The listing builds one solid part. Answer for the finished solid, in the listing's coordinates (mm). Face numbers are marked on the shaded views. A direction names the side the tool comes from. Give positions to 0.01 mm unless a question says otherwise; leave off trailing zeros. Write each loop counter-clockwise with the first axis right and the second up, starting at its lowest first coordinate (ties: lowest second). Pieces come first, ordered by that corner, then holes. Notation, with made-up numbers: (9.5, -39.75) - (36.5, -39.75) arc R15 ccw to (36.5, -10.75) - close; hole circle Ø3 at (20.5, 11.5). An arc over 180 degrees is marked (long way). One line per item, written item: value. Start each with the question number.
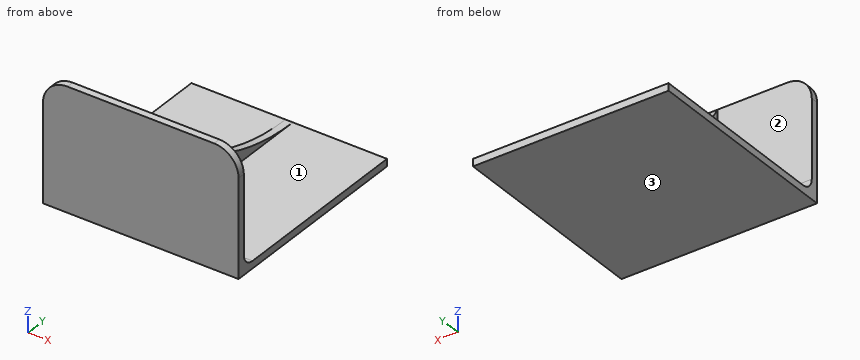
from build123d import *

# Parameters (mm, degrees)
SKETCH1_W           = 80
SKETCH1_H           = 50
BOSS_EXTRUDE1_DEPTH = 3
SKETCH2_W           = 80
SKETCH2_H           = 3
BOSS_EXTRUDE2_DEPTH = 82
BOSS_EXTRUDE3_DEPTH = 1.5
FILLET1_R           = 10
FILLET2_R           = 5


with BuildPart() as part:
    # Sketch1 → Boss-Extrude1 (new body)
    with BuildSketch(Plane(origin=(0, 0, 0), x_dir=(1, 0, 0), z_dir=(0, 1, 0))):
        Rectangle(SKETCH1_W, SKETCH1_H)
    extrude(amount=BOSS_EXTRUDE1_DEPTH)

    # Sketch2 → Boss-Extrude2 (add)
    with BuildSketch(Plane(origin=(0, 3, 0), x_dir=(1, 0, 0), z_dir=(0, 1, 0))):
        with Locations((0, 23.5)):
            Rectangle(SKETCH2_W, SKETCH2_H)
    extrude(amount=BOSS_EXTRUDE2_DEPTH)

    # Sketch3 → Boss-Extrude3 (add, symmetric)
    with BuildSketch(Plane(origin=(0, 0, 0), x_dir=(0, 0, -1), z_dir=(1, 0, 0))):
        with BuildLine():
            Line((22, 85), (22, 3))
            Line((22, 3), (-25, 3))
            ThreePointArc((-25, 3), (9.416947126, 37.742725428), (22, 85))
        make_face()
    extrude(amount=BOSS_EXTRUDE3_DEPTH, both=True)

    # Fillet1
    fillet1_edges = [part.edges().sort_by_distance(p)[0] for p in [
        (40, 1.5, 25),
        (-40, 1.5, 25),
    ]]
    fillet(fillet1_edges, radius=FILLET1_R)

    # Fillet2
    fillet2_edges = [part.edges().sort_by_distance(p)[0] for p in [
        (-20.75, 3, -22),
        (20.75, 3, -22),
    ]]
    fillet(fillet2_edges, radius=FILLET2_R)


solid = part.part
Item 1: Find section C-C on z = -9. Determine the outline of the cut face in (x, y).
Item 2: Each of these flat-tipped pins is pushed along its axis until it touches: pin 1 Ø23.5 at (y, z) = (27.5, 3) entering from +X; pin 2 Ø19 at (x, y) = (29, 37.5) entering from +Z. Where does it stop, or does it pass through?
Item 3: For the marked faces 1, 2 and 3, determine the directions among +Z, -Z, +X, -X, +Y, -Y from which every point of the face is accessible in a straight line to the end or side of a thin tool.
Item 4: Straight lines are drawn through the part: line 1 along Y through (x, z) = (35, -7); line 2 along Z through (x, y) = (35.5, 26); line 3 along X through (y, z) = (9, -6.5). For each, find the intervals that lie inside material, in ascending order.
Item 5: Find section A-A on y = 61.5. Determine the outline of the cut face in (x, z).
Item 6: Find section B-B on x = -19. Determine the outline of the cut face in (y, z), plus the area to 3 significant figures.
Values:
1. outline: (-40, 0) - (40, 0) - (40, 3) - (1.5, 3) - (1.5, 37.02) - (-1.5, 37.02) - (-1.5, 3) - (-40, 3) - close
2. pin 1: x = 1.5
2. pin 2: z = -22
3. face 1: +Z, +X, +Y
3. face 2: +Z, -X, +Y
3. face 3: -Z, +X, -X, +Y, -Y
4. line 1: 0 to 3
4. line 2: -25 to -22
4. line 3: -1.5 to 1.5
5. outline: (-40, -25) - (40, -25) - (40, -22) - (1.5, -22) - (1.5, -19.05) - (-1.5, -19.05) - (-1.5, -22) - (-40, -22) - close
6. outline: (0, -25) - (85, -25) - (85, -22) - (8, -22) arc R5 cw to (3, -17) - (3, 25) - (0, 25) - close
6. area: 401 mm^2
